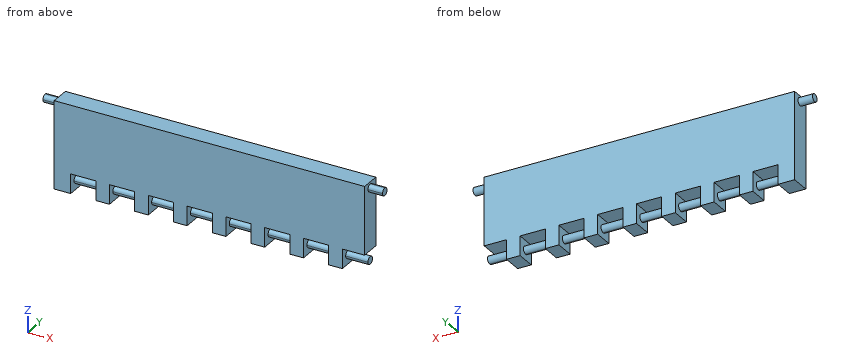
```python
from build123d import *

# Parameters (mm, degrees)
F0_W          = 17.78
F0_H          = 25.4
F0_W_2        = 3.81
F1_DEPTH      = 25.4
F3_DEPTH      = 406.4
F5_DEPTH      = 19.05
F5_DEPTH_BACK = 425.45


with BuildPart() as f1:
    # F0 (on Front) → F1 (new body)
    with BuildSketch(Plane.XZ):
        Polygon((199.39, -31.75), (203.2, -31.75), (203.2, 57.15), (-203.2, 57.15), (-203.2, -31.75), (-199.39, -31.75), (-181.61, -31.75), (-177.8, -31.75), (-173.99, -31.75), (-156.21, -31.75), (-152.4, -31.75), (-148.59, -31.75), (-130.81, -31.75), (-127, -31.75), (-123.19, -31.75), (-105.41, -31.75), (-101.6, -31.75), (-97.79, -31.75), (-80.01, -31.75), (-76.2, -31.75), (-72.39, -31.75), (-54.61, -31.75), (-50.8, -31.75), (-46.99, -31.75), (-29.21, -31.75), (-25.4, -31.75), (-21.59, -31.75), (-3.81, -31.75), (0, -31.75), (3.81, -31.75), (21.59, -31.75), (25.4, -31.75), (29.21, -31.75), (46.99, -31.75), (50.8, -31.75), (54.61, -31.75), (72.39, -31.75), (76.2, -31.75), (80.01, -31.75), (97.79, -31.75), (101.6, -31.75), (105.41, -31.75), (123.19, -31.75), (127, -31.75), (130.81, -31.75), (148.59, -31.75), (152.4, -31.75), (156.21, -31.75), (173.99, -31.75), (177.8, -31.75), (181.61, -31.75), align=None)
        with Locations((-190.5, -44.45)):
            Rectangle(F0_W, F0_H)
        with Locations((-139.7, -44.45)):
            Rectangle(F0_W, F0_H)
        with Locations((-88.9, -44.45)):
            Rectangle(F0_W, F0_H)
        with Locations((-38.1, -44.45)):
            Rectangle(F0_W, F0_H)
        with Locations((12.7, -44.45)):
            Rectangle(F0_W, F0_H)
        with Locations((63.5, -44.45)):
            Rectangle(F0_W, F0_H)
        with Locations((165.1, -44.45)):
            Rectangle(F0_W, F0_H)
        with Locations((114.3, -44.45)):
            Rectangle(F0_W, F0_H)
        with Locations((-201.295, -44.45)):
            Rectangle(F0_W_2, F0_H)
    extrude(amount=F1_DEPTH)

    # F2 (on face) → F3 (join)
    with BuildSketch(Plane(origin=(-203.2, 0, 0), x_dir=(0, -1, 0), z_dir=(-1, 0, 0))):
        with BuildLine():
            ThreePointArc((12.7, -49.53), (16.292102, -48.042102), (17.78, -44.45))
            ThreePointArc((17.78, -44.45), (9.107898, -40.857898), (12.7, -49.53))
        make_face()
    extrude(amount=-F3_DEPTH)

    # F4 (on face) → F5 (join, two sides)
    with BuildSketch(Plane(origin=(-203.2, 0, 0), x_dir=(0, -1, 0), z_dir=(-1, 0, 0))) as f5_sk:
        with BuildLine():
            ThreePointArc((12.7, 54.61), (9.107898, 45.937898), (17.78, 49.53))
            ThreePointArc((17.78, 49.53), (16.292102, 53.122102), (12.7, 54.61))
        make_face()
    extrude(amount=F5_DEPTH)
    extrude(f5_sk.sketch, amount=-F5_DEPTH_BACK)


solid = f1.part
```
The listing builds one solid part. Answer for the finished solid, in the listing's coordinates (mm). Give positions to 0.01 mm unless a question says otherwise; leave off trailing zeros. Loops run counter-clockwise (first coordinate to the right, second up) from the corner with the lowest first, then second, coordinate; pieces in that order, holes last. Notation, with made-up numbers: (75.5, -26) - (80.5, -26) arc R24 cw to (80.5, -10) - close; hole circle Ø6 at (-0.5, 70). An arc over 180 degrees is marked (long way). Return JSON: item names as keys, results as strings. Group by question number.
1. Straight lines are drawn through the part: line 1 (X direction, y = -19.5, z = 14); line 2 (Z direction, x = -54, y = -16.5); line 3 (Z direction, x = 138, y = -15). For each, find the intervals that lie inside material, in ascending order. Write a range as [from, to].
2. Find section A-A (x = -159). Write down the section's boundary in (y, z).
3. Given pin 1 Ø7.5 at (x, y) = (87, -16.5) entering from -Z; pin 2 Ø12.5 at (y, z) = (-14, -50) entering from +X; pin 3 Ø7.5 at (y, z) = (-14, -46.5) entering from -X, each flat-ended and moving along its own axis, determine where each tip first touches the part or whether it passes through.
4. Find section B-B (z = 15). Write down the section's boundary in (x, y).
Verdict:
{
 "1": {"line 1": "x = [-203.2, 203.2]", "line 2": "z = [-47.82, -41.08], [-31.75, 57.15]", "line 3": "z = [-48.98, -39.92], [-31.75, 57.15]"},
 "2": {"outline": "(-25.4, -31.75) - (0, -31.75) - (0, 57.15) - (-25.4, 57.15) - close; (-17.78, -44.45) arc R5.08 ccw to (-12.7, -49.53) arc R5.08 ccw (long way) to start"},
 "3": {"pin 1": "stops at z = -49.53", "pin 2": "stops at x = 203.2", "pin 3": "stops at x = -203.2"},
 "4": {"outline": "(-203.2, -25.4) - (203.2, -25.4) - (203.2, 0) - (-203.2, 0) - close"}
}
